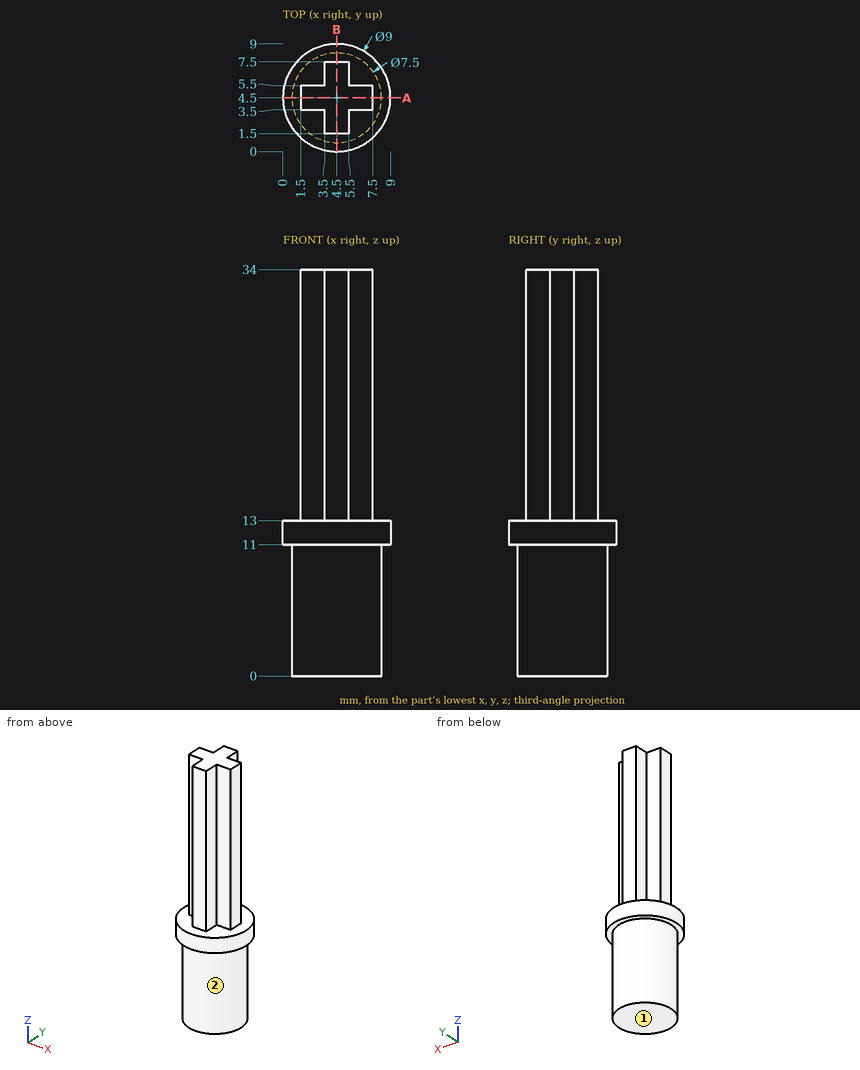
Geometry check sheet. Reference: drawing and pictorial views, mm from the part's lowest x, y, z. A direction names the side the tool comes from. Round coordinates to 2 decimals unless told otherwise and drop trailing zeros. Order: outer loops, then holes, each group sorted by start corner. A loop starts at its lowest first (then second) coordinate and runs counter-clockwise, first axis right, second up. Notation, with made-up numbers: (-28.75, -10.75) -> (-21.75, -10.75) arc R16 cw to (-21.75, -0.75) -> close; hole circle Ø4 at (-27.5, 17.25). An arc over 180 degrees is marked (long way). One line per item, written item: value. Start each with the question number.
Q1. Gauge pin test, flat ends, axial feed: pin 1 Ø1.6 at (x, z) = (6, 19) entering from +Y; pin 2 Ø0.6 at (y, z) = (2, 27.5) entering from -X; pin 3 Ø1.6 at (y, z) = (7, 19.5) entering from +X. Record the tip position at first contact, or that the pin passes through.
Q2. Thickness scan on line 1 (Z direction, x = 3, y = 1); line 2 (X direction, y = 3.25, z = 22.5); line 3 (Z direction, x = 3.75, y = 1). Record the ranges inside material, lowest first.
Q3. Set-up check for the marked faces 1 and 2: record each of +Z, -Z, +X, -X, +Y, -Y from which the full face is reachable in a straight line by a thin tool's end or side.
Q4. Cross-section at A-A (y = 4.5). Record the boundary of the cut face in (x, z).
Completed:
1. pin 1: stops at y = 7.5
1. pin 2: stops at x = 3.5
1. pin 3: stops at x = 5.5
2. line 1: z = 11 to 13
2. line 2: x = 3.5 to 5.5
2. line 3: z = 0 to 13
3. face 1: -Z, +X, -X, +Y, -Y
3. face 2: -Z
4. outline: (0, 11) -> (0.75, 11) -> (0.75, 0) -> (8.25, 0) -> (8.25, 11) -> (9, 11) -> (9, 13) -> (7.5, 13) -> (7.5, 34) -> (1.5, 34) -> (1.5, 13) -> (0, 13) -> close
